from build123d import *

# Parameters (mm, degrees)
F0_W     = 20
F0_H     = 20
F1_DEPTH = 20
F2_R     = 2
F4_DEPTH = 1
F3_R     = 2
F5_DEPTH = 1
F6_R     = 2
F7_DEPTH = 1
F8_R     = 2
F9_DEPTH = 1


with BuildPart() as f1:
    # F0 (on Top) → F1 (new body)
    with BuildSketch(Plane.XY):
        with Locations((-10, 10)):
            Rectangle(F0_W, F0_H)
    extrude(amount=F1_DEPTH)

    # F2 (on face) → F4 (cut)
    with BuildSketch(Plane.XY.offset(20)):
        with Locations((-10, 10)):
            Circle(F2_R)
    extrude(amount=-F4_DEPTH, mode=Mode.SUBTRACT)

    # F3 (on face) → F5 (cut)
    with BuildSketch(Plane.YZ):
        with Locations((15, 5)):
            Circle(F3_R)
        with Locations((5, 15)):
            Circle(F3_R)
    extrude(amount=-F5_DEPTH, mode=Mode.SUBTRACT)

    # F6 (on face) → F7 (cut)
    with BuildSketch(Plane(origin=(0, 20, 0), x_dir=(-1, 0, 0), z_dir=(0, 1, 0))):
        with Locations((15, 5)):
            Circle(F6_R)
        with Locations((5, 5)):
            Circle(F6_R)
        with Locations((5, 15)):
            Circle(F6_R)
        with Locations((15, 15)):
            Circle(F6_R)
    extrude(amount=-F7_DEPTH, mode=Mode.SUBTRACT)

    # F8 (on face) → F9 (cut)
    with BuildSketch(Plane(origin=(-20, 0, 0), x_dir=(0, -1, 0), z_dir=(-1, 0, 0))):
        with Locations((-10, 10)):
            Circle(F8_R)
        with Locations((-5, 15)):
            Circle(F8_R)
        with Locations((-5, 5)):
            Circle(F8_R)
        with Locations((-15, 5)):
            Circle(F8_R)
        with Locations((-15, 15)):
            Circle(F8_R)
    extrude(amount=-F9_DEPTH, mode=Mode.SUBTRACT)


solid = f1.part
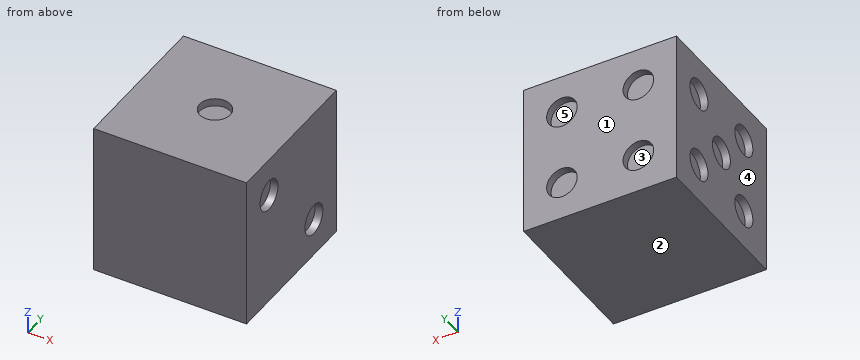
Design review of the part built by this model. Coordinates are the model's own, in mm. Face numbers are marked on the shaded views. A direction names the side the tool comes from. Give positions to 0.01 mm unless a question says otherwise; leave off trailing zeros. Write each loop counter-clockwise with the first axis right and the second up, starting at its lowest first coordinate (ties: lowest second). Pieces come first, ordered by that corner, then holes. Notation, with made-up numbers: M 68,-1 L 100,-1 A16 ccw 100,4 Z; hole C 14.25,15 d9. An arc over 180 degrees is marked long. Return JSON: item names as keys, results as strings. Group by question number.
Item 1: Take a section at C-C (z = 6). Give the boundary of the cut face in (x, y), plus the area to 3 significant figures.
Item 2: Clearance check with flat-ended pins moving along their axes: pin 1 Ø1.2 at (y, z) = (5.5, 15.5) entering from +X; pin 2 Ø1.2 at (y, z) = (15.5, 5) entering from -X; pin 3 Ø1.2 at (x, z) = (-5.5, 15.5) entering from +Y. State where each tip first meets the part, or that it passes through.
Item 3: Take a section at A-A (y = 5). Give the boundary of the cut face in (x, z), plus the area to 3 significant figures.
Item 4: Tool access review of the marked faces 4 and 5: name each direction out of +Z, -Z, +X, -X, +Y, -Y from which nothing blocks a thin tool from reaching the whole face with its end or side.
Item 5: Take a section at B-B (x = -5). Give the boundary of the cut face in (y, z).
Item 6: Wall thickness on line 1 along Z through (x, y) = (-15, 19.8); line 2 along Z through (x, y) = (-19.35, 10); line 3 along X through (y, z) = (5.5, 5.75): over which ranges is each line inside the solid? List them lowest first.
Item 7: The part is to be moulded in two halves that separate along Z. For the marked faces 1, 2 and 3, say which applies: pulls with the +Z half, pulls with the -Z half, needs draft (parallel to the pull), parting line crosses it, or undercut.
Item 8: Take a section at D-D (y = 15.75). Give the boundary of the cut face in (x, z).
Return value:
{
 "1": {"outline": "M -20,0 L 0,0 L 0,13.27 L -1,13.27 L -1,16.73 L 0,16.73 L 0,20 L -3.27,20 L -3.27,19 L -6.73,19 L -6.73,20 L -13.27,20 L -13.27,19 L -16.73,19 L -16.73,20 L -20,20 L -20,16.73 L -19,16.73 L -19,13.27 L -20,13.27 L -20,6.73 L -19,6.73 L -19,3.27 L -20,3.27 Z", "area": "383 mm2"},
 "2": {"pin 1": "stops at x = -1", "pin 2": "stops at x = -19", "pin 3": "stops at y = 19"},
 "3": {"outline": "M -20,0 L 0,0 L 0,13 L -1,13 L -1,17 L 0,17 L 0,20 L -20,20 L -20,17 L -19,17 L -19,13 L -20,13 L -20,7 L -19,7 L -19,3 L -20,3 Z", "area": "388 mm2"},
 "4": {"face 4": "+Z, -Z, -X, +Y, -Y", "face 5": "+Y"},
 "5": {"outline": "M 0,0 L 20,0 L 20,3 L 19,3 L 19,7 L 20,7 L 20,13 L 19,13 L 19,17 L 20,17 L 20,20 L 0,20 Z"},
 "6": {"line 1": "z = 0 to 3, 7 to 13, 17 to 20", "line 2": "z = 0 to 8, 12 to 20", "line 3": "x = -19 to 0"},
 "7": {"face 1": "needs draft", "face 2": "pulls with the -Z half", "face 3": "undercut"},
 "8": {"outline": "M -20,0 L 0,0 L 0,3.15 L -1,3.15 L -1,6.85 L 0,6.85 L 0,20 L -20,20 L -20,16.85 L -19,16.85 L -19,13.15 L -20,13.15 L -20,6.85 L -19,6.85 L -19,3.15 L -20,3.15 Z"}
}
